Input: dimensioned drawing with shaded views. Units: mm. Origin: part minimum x, y, z. A direction names the side the tool comes from. Give positions to 0.01 mm unless a question says otherwise; leave off trailing zeros. Write each loop counter-clockwise with the first axis right and the second up, starting at its lowest first coordinate (ties: lowest second). Pieces come first, ordered by that corner, then holes. Notation, with made-up numbers: (32, 59) -> (80, 59) arc R21 ccw to (80, 94) -> close; hole circle Ø10 at (-1, 60). An arc over 180 degrees is marked (long way). Answer as a JSON object with one key per item and string values. Group by question number.
(1) Set-up query: the marked faces 1, 2 and 3. Return all of +Z, -Z, +X, -X, +Y, -Y with unobstructed straight access to the full face (end or side cutting, diameter ignored); none if empty.
(2) Section query D-D on y = 31. Output: boundary loops of the cut face in (x, z).
(3) Section query A-A on y = 13. Output: boundary loops of the cut face in (x, z), plus the area to 3 significant figures.
(4) Contact query for flat-ended pins moving along their axis: pin 1 Ø2 at (y, z) = (44.5, 82) entering from -X; pin 2 Ø6 at (x, y) = (16.5, 42.5) entering from -Z; pin 3 Ø14.5 at (x, z) = (11.5, 45) entering from +Y. Output: stop coordinate, or through.
(5) Section query C-C on z = 13. Output: boundary loops of the cut face in (x, y).
(6) Section query B-B on x = 6.5. Output: boundary loops of the cut face in (y, z), plus the area to 3 significant figures.
(7) Material intervals for probe 1 along Z at (x, y) = (24, 55.5); probe 2 along X at (y, z) = (4, 32.5); probe 3 along Y at (x, z) = (26, 47.5), sorted ascending.
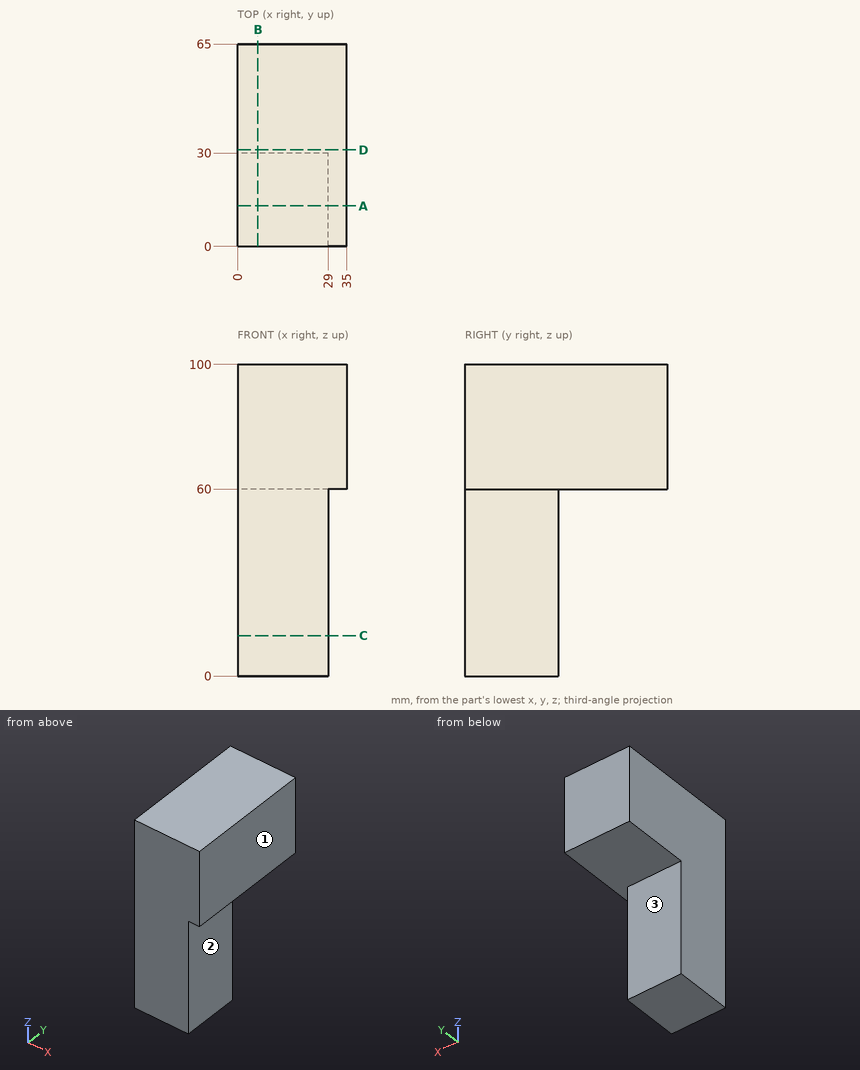
Answer list:
{
 "1": {"face 1": "+Z, -Z, +X, +Y, -Y", "face 2": "-Z, +X, +Y, -Y", "face 3": "-Z, +X, -X, +Y"},
 "2": {"outline": "(0, 60) -> (35, 60) -> (35, 100) -> (0, 100) -> close"},
 "3": {"outline": "(0, 0) -> (29, 0) -> (29, 60) -> (35, 60) -> (35, 100) -> (0, 100) -> close", "area": "3,140 mm2"},
 "4": {"pin 1": "x = 0", "pin 2": "z = 60", "pin 3": "y = 30"},
 "5": {"outline": "(0, 0) -> (29, 0) -> (29, 30) -> (0, 30) -> close"},
 "6": {"outline": "(0, 0) -> (30, 0) -> (30, 60) -> (65, 60) -> (65, 100) -> (0, 100) -> close", "area": "4,400 mm2"},
 "7": {"probe 1": "60 to 100", "probe 2": "0 to 29", "probe 3": "0 to 30"}
}
